Design review of the part shown in the three views and the two pictorial views. Dimensions are in mm from the part's minimum x, y and z. A direction names the side the tool comes from. Round coordinates to 2 decimals unless told otherwise and drop trailing zeros. Loops run counter-clockwise (first coordinate to the right, second up) from the corner with the lowest first, then second, coordinate; pieces in that order, holes last. Notation, with made-up numbers: (84.5, 84) -> (122.5, 84) arc R23 ccw to (122.5, 97) -> close; hole circle Ø8 at (10, 64.25). An arc over 180 degrees is marked (long way). Write each question's results on one line, items separated by ' | '. Start each with the question number.
Item 1: We need section B-B (z = 24.5). Give the boundary of the cut face in (x, y), and give its area (4 significant figures).
Item 2: We need section D-D (y = 18). Give the boundary of the cut face in (x, z).
Item 3: We need section C-C (y = 3). Give the boundary of the cut face in (x, z).
Item 4: We need section A-A (x = 24.5). Give the boundary of the cut face in (y, z), and give its area (4 significant figures).
Item 5: Tool access review of the marked faces 1 and 2: name each direction out of +Z, -Z, +X, -X, +Y, -Y from which nothing blocks a thin tool from reaching the whole face with its end or side.
Item 6: For L1, parallel to Y at x = 37, z = 6; L2, parallel to Z at x = 24, y = 14; L3, parallel to Z at x = 29, y = 20.5, list the stretches that pass through material, from the lowest coordinate up. Write a range as from..to.
Item 7: Clearance check with flat-ended pins moving along their axes: pin 1 Ø8 at (x, y) = (19, 25.5) entering from +Z; pin 2 Ø10 at (x, y) = (19.5, 8.5) entering from -Z; pin 3 Ø5 at (y, z) = (15.5, 9.5) entering from -X. State where each tip first meets the part, or that it passes through.
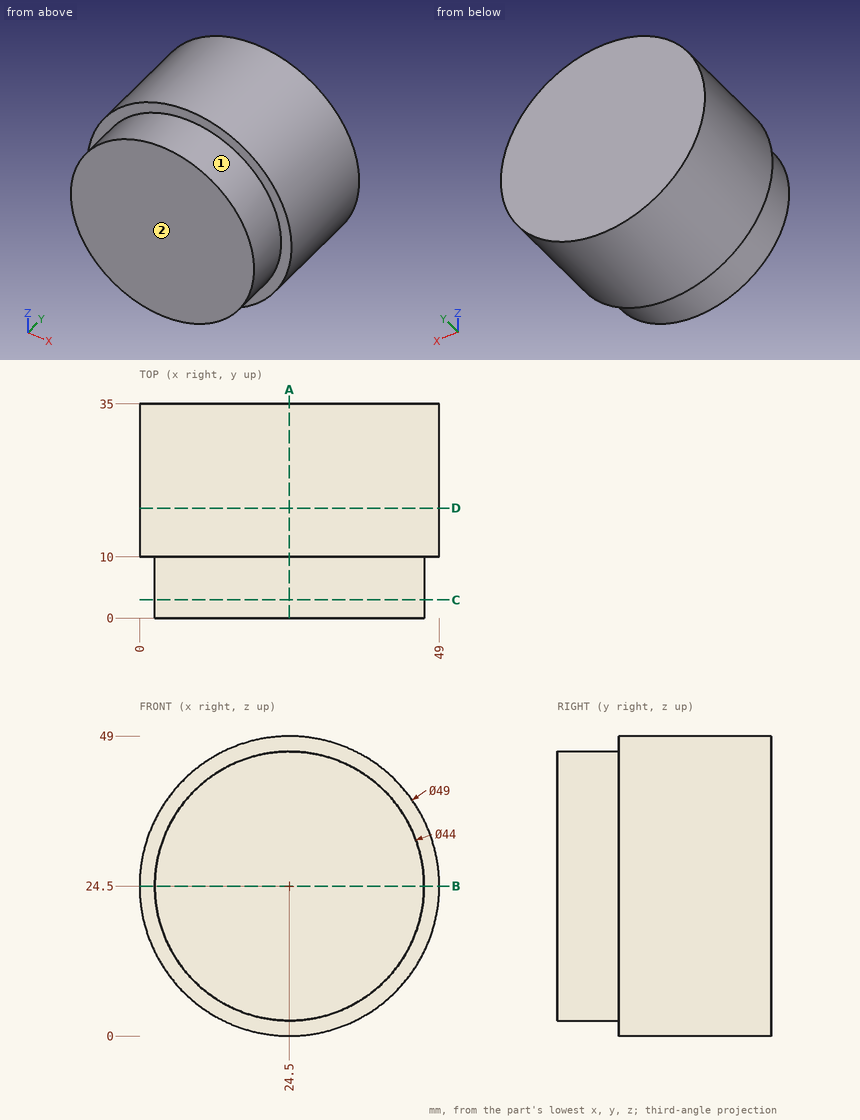
Here are the results:
1) outline: (0, 10) -> (2.5, 10) -> (2.5, 0) -> (46.5, 0) -> (46.5, 10) -> (49, 10) -> (49, 35) -> (0, 35) -> close | area: 1,665 mm2
2) outline: circle Ø49 at (24.5, 24.5)
3) outline: circle Ø44 at (24.5, 24.5)
4) outline: (0, 2.5) -> (10, 2.5) -> (10, 0) -> (35, 0) -> (35, 49) -> (10, 49) -> (10, 46.5) -> (0, 46.5) -> close | area: 1,665 mm2
5) face 1: -Y | face 2: +Z, -Z, +X, -X, -Y
6) L1: y = 10..35 | L2: z = 0.01..48.99 | L3: z = 0.42..48.58
7) pin 1: stops at z = 48.95 | pin 2: stops at z = 0 | pin 3: stops at x = 3.43
